Autodesk Inventor part; units mm, degrees
ref_plane "YZ Plane" through (0, 0, 0) normal (1, 0, 0) x (0, 1, 0)
ref_plane "XZ Plane" through (0, 0, 0) normal (0, 1, 0) x (-1, 0, 0)
ref_plane "XY Plane" through (0, 0, 0) normal (0, 0, 1) x (1, 0, 0)
sketch "Szkic1" plane through (0, 0, 0) normal (0, 0, 1) x (1, 0, 0)
  line L0 (0, 0) -> (36, 0)
  line L1 (36, 0) -> (36, 36)
  line L2 (36, 36) -> (0, 36)
  line L3 (0, 36) -> (0, 0)
  line L4 (0, 0) -> (-24, 0)
  line L5 (-42, 18) -> (-42, 18)
  line L6 (-42, 18) -> (0, 18)
  line L7 (0, 18) -> (0, 0)
  line L8 (36, 36) -> (78, 36)
  line L9 (78, 36) -> (78, 32)
  line L10 (46, 0) -> (36, 0)
  line L11 (36, 0) -> (36, 36)
  line L12 (78, 36) -> (48, 36)
  line L13 (48, 36) -> (48, 76)
  line L14 (48, 76) -> (78, 76)
  line L15 (78, 76) -> (78, 36)
  arc A0 (46, 0) -> (78, 32) centre (46, 32) ccw
  arc A1 (-42, 18) -> (-24, 0) centre (-24, 18) ccw
  point P0 (-42, 0)
  point P1 (78, 0)
  dimension "d0" = 36
  dimension "d1" = 36
  dimension "d2" = 42
  dimension "d3" = 18
  dimension "d4" = 42
  dimension "d5" = 30
  dimension "d6" = 40
  dimension "d7" = 32
  dimension "d8" = 18
extrude "Wyciągnięcie proste1" add sketch "Szkic1" against normal blind 24
sketch "Szkic2" plane through (0, 0, 0) normal (0, 0, 1) x (1, 0, 0)
  line L0 (78, 76) -> (78, 32)
  line L1 (46, 0) -> (-24, 0)
  line L2 (78, 76) -> (36, 76)
  line L3 (36, 76) -> (36, 0)
  line L4 (36, 0) -> (78, 0)
  line L5 (78, 0) -> (78, 76)
  point P0 (0, 0)
extrude "Wyciągnięcie proste2" cut sketch "Szkic2" against normal blind 3
sketch "Szkic3" plane through (0, 0, -24) normal (0, 0, -1) x (-1, 0, 0)
  line L0 (-48, 76) -> (-78, 76)
  line L1 (-46, 0) -> (-36, 0)
  line L2 (-78, 76) -> (-36, 76)
  line L3 (-36, 76) -> (-36, 0)
  line L4 (-36, 0) -> (-78, 0)
  line L5 (-78, 0) -> (-78, 76)
  line L6 (0, 36) -> (0, 18)
  line L7 (0, 36) -> (42, 36)
  line L8 (42, 36) -> (42, 0)
  line L9 (42, 0) -> (0, 0)
  line L10 (0, 0) -> (0, 36)
  point P0 (0, 0)
extrude "Wyciągnięcie proste3" cut sketch "Szkic3" against normal blind 9 contours L2 L3 L1 L4 L5 L0
sketch "Szkic4" plane through (0, 0, -24) normal (0, 0, -1) x (-1, 0, 0)
  line L0 (42, 18) -> (0, 18)
  line L1 (0, 0) -> (42, 0)
  line L2 (42, 0) -> (42, 18)
  line L3 (42, 18) -> (0, 18)
  line L4 (0, 18) -> (0, 0)
extrude "Wyciągnięcie proste4" cut sketch "Szkic4" against normal blind 9
ref_plane "Płaszczyzna konstrukcyjna1" through (-42, 18, 0) normal (-1, 0, 0) x (0, -1, 0)
sketch "Szkic5" plane through (-42, 18, 0) normal (-1, 0, 0) x (0, -1, 0)
  line L0 (0, 0) -> (0, -15)
  line L1 (-18, -15) -> (18, -15)
  line L2 (0, -15) -> (-16, -43.6236)
  line L3 (-16, -43.6236) -> (-37, -43.6236)
  line L4 (-37, -43.6236) -> (-37, -28.6236)
  line L5 (-37, -28.6236) -> (-20, -28.6236)
  line L6 (-20, -28.6236) -> (-4, 0)
  line L7 (-18, 0) -> (0, 0)
  line L8 (0, 0) -> (0, -15)
  point P0 (18, 0)
  point P1 (-28.5, -28.6236)
  dimension "d17" = 16
  dimension "d18" = 15
  dimension "d19" = 4
  dimension "d20" = 16
  dimension "d21" = 21
extrude "Wyciągnięcie proste5" add sketch "Szkic5" against normal blind 18
full round fillet "Zaokrąglenie pełne1" first side at (-24, 26, -14.5412) centre faces at (-36, 55, -33.6236) second side at (-42, 26, -14.5412)
sketch "Szkic6" plane through (-42, 38, -28.6236) normal (0, 0, 1) x (1, 0, 0)
  arc A0 (18, 8) -> (0, 8) centre (9, 8) ccw
  point P0 (42, -38)
hole "Otwór1" at (-33, 46, -28.6236) direction (0, 0, -1) diameter 9 end through all
sketch "Szkic7" plane through (48, 36, -3) normal (-1, 0, 0) x (0, 0, 1)
  point P0 (3, -36)
  point P1 (-6, 34)
hole "Otwór2" at (48, 70, -9) direction (1, 0, 0) diameter 6 end through all
sketch "Szkic8" plane through (0, 0, -3) normal (0, 0, 1) x (1, 0, 0)
  point P0 (0, 0)
  point P1 (63, 52)
hole "Otwór3" at (63, 52, -3) direction (0, 0, -1) diameter 18 end through all
sketch "Szkic9" plane through (48, 76, -3) normal (0, 1, 0) x (1, 0, 0)
  line L0 (0, 0) -> (30, 0)
  line L1 (14, 12) -> (16, 12)
  line L2 (16, 12) -> (16, 0)
  line L3 (16, 0) -> (14, 0)
  line L4 (14, 0) -> (14, 12)
  line L5 (30, 0) -> (30, 12)
  point P0 (-48, -3)
  point P1 (14, 0)
  dimension "d45" = 2
  dimension "d46" = 14
extrude "Wyciągnięcie proste6" cut sketch "Szkic9" against normal up to surface
sketch "Szkic10" plane through (0, 36, 0) normal (0, 1, 0) x (1, 0, 0)
  line L0 (6, 18) -> (30, 18)
  line L1 (30, 18) -> (30, 6)
  line L2 (30, 6) -> (6, 6)
  line L3 (6, 6) -> (6, 18)
  line L4 (0, 24) -> (36, 24)
  line L5 (0, 0) -> (0, 24)
  point P0 (6, 12)
  dimension "d49" = 24
  dimension "d50" = 12
  dimension "d51" = 6
  dimension "d52" = 6
extrude "Wyciągnięcie proste7" cut sketch "Szkic10" against normal through all
CAD build for the part. Positions are in the model's coordinates, mm. A direction names the side the tool comes from. Coordinates: 2 decimals unless noted, no trailing zeros. Loops run counter-clockwise (first coordinate to the right, second up) from the corner with the lowest first, then second, coordinate; pieces in that order, holes last. Notation, with made-up numbers: (54.5, 22.25) - (68.5, 22.25) arc R32 ccw to (68.5, 58.25) - close; hole circle Ø7 at (74, 33). An arc over 180 degrees is marked (long way). Write item = value, one per line. Start each with the question number.
Q1. Cut at A-A, the plane x = 28.5. List the corners of the cut face in (y, z).
Q2. Cut at B-B, the plane y = 70. List the corners of the cut face in (x, z).
Q3. Cut at D-D, the plane y = 40. List the corners of the cut face in (x, z).
Q4. Pull direction Y, two halves, no side cores. Call faces 4 (the flat face through (48, 56, -9)), 5 (the flat face through (-33.126, 25.888, -29.111)), 6 (the cylindrical face through (71.1, 72.93, -9.65)), 7 (the cylindrical face through (55.1, 72.93, -9.65)): pulls with the +Y half, pulls with the -Y half, needs draft (parallel to the pull), parting line crosses it, or undercut.
Q5. Cut at C-C, the plane x = 56. List the corners of the cut face in (y, z).
Q6. Flat gauge pins, fed straight in: pin 1 Ø2.5 at (y, z) = (11, -1.5) entering from +X; pin 2 Ø19 at (x, z) = (23.5, -9.5) entering from +Y; pin 3 Ø12.5 at (x, y) = (61.5, 55) entering from +Z. Where does each tip first touch, or does it go through?
Q7. Which spindle directions (+Z, -Z, +X, -X, +Y, -Y) get a long thin tool onto all of the face, cutting with end or side? Do faces 1 (the flat face through (36, 18, -20)), 2 (the flat face through (18, 18, -6)), 3 (the flat face through (24, 36, -4)). Say none if no direction does.
Q8. Drill centre lines: L1, parallel to Z at x = 23, y = 28.5; L2, parallel to Y at x = 59, z = -9; L3, parallel to X at y = 30, z = -17.5. Where is each one in solid material? Low to high.
Computed:
q1.outline = (0, -24) - (36, -24) - (36, -18) - (0, -18) - close; (0, -6) - (36, -6) - (36, 0) - (0, 0) - close
q2.outline = (48, -15) - (62, -15) - (62, -12) - (48, -12) - close; (48, -6) - (62, -6) - (62, -3) - (48, -3) - close; (64, -15) - (78, -15) - (78, -12) - (64, -12) - close; (64, -6) - (78, -6) - (78, -3) - (64, -3) - close
q3.outline = (-42, -43.62) - (-24, -43.62) - (-24, -28.62) - (-42, -28.62) - close; (48, -15) - (78, -15) - (78, -3) - (48, -3) - close
q4.face_4 = needs draft
q4.face_5 = pulls with the -Y half
q4.face_6 = undercut
q4.face_7 = undercut
q5.outline = (1.6, -15) - (46.34, -15) - (46.34, -3) - (1.6, -3) - close; (57.66, -15) - (76, -15) - (76, -3) - (57.66, -3) - close; hole circle Ø6 at (70, -9)
q6.pin_1 = 36
q6.pin_2 = 36
q6.pin_3 = -3
q7.face_1 = -Z, +X, +Y, -Y
q7.face_2 = +Y, -Y
q7.face_3 = +Z, -Z, -X, +Y
q8.L1 = -24 to -18, -6 to 0
q8.L2 = 2.76 to 43.94, 60.06 to 67, 73 to 76
q8.L3 = -42 to -24, 0 to 6, 30 to 36
